from build123d import *

# Parameters (mm, degrees)
F1_R      = 60.325
F2_DEPTH  = 127
F0_R      = 53.975
F3_DEPTH  = 184.912
F5_DEPTH  = 19.05
F6_R      = 1.5875
F7_DEPTH  = 25.4
F8_R      = 1.5875
F9_DEPTH  = 25.4
F10_R     = 1.5875
F11_DEPTH = 36.6522


with BuildPart() as f2:
    # F1 (on Top) → F2 (new body)
    with BuildSketch(Plane.XY):
        Circle(F1_R)
    extrude(amount=F2_DEPTH)

    # F0 (on Top) → F3 (cut)
    with BuildSketch(Plane.XY):
        Circle(F0_R)
    extrude(amount=F3_DEPTH, mode=Mode.SUBTRACT)

    # F4 (on Top) → F5 (join)
    with BuildSketch(Plane.XY):
        with BuildLine():
            ThreePointArc((-56.3123252778, 21.5134135298), (-55.0938321912, 24.4657841564), (-53.7206778829, 27.3494736274))
            Line((-53.7206778829, 27.3494736274), (-67.5786357684, 35.350369343))
            Line((-67.5786357684, 35.350369343), (-70.7536357684, 29.851108029))
            Line((-70.7536357684, 29.851108029), (-56.3123252778, 21.5134135298))
        make_face()
        with BuildLine():
            Line((-64.4036357684, 40.849630657), (-50.5456778829, 32.8487349414))
            ThreePointArc((-50.5456778829, 32.8487349414), (-48.7349066985, 35.4797661912), (-46.7873252778, 38.0111974719))
            Line((-46.7873252778, 38.0111974719), (-61.2286357684, 46.348891971))
            Line((-61.2286357684, 46.348891971), (-64.4036357684, 40.849630657))
        make_face()
        with BuildLine():
            Line((67.5786357684, 35.350369343), (53.7206778829, 27.3494736274))
            ThreePointArc((53.7206778829, 27.3494736274), (55.0938321912, 24.4657841564), (56.3123252778, 21.5134135298))
            Line((56.3123252778, 21.5134135298), (70.7536357684, 29.851108029))
            Line((70.7536357684, 29.851108029), (67.5786357684, 35.350369343))
        make_face()
        with BuildLine():
            ThreePointArc((46.7873252778, 38.0111974719), (48.7349066985, 35.4797661912), (50.5456778829, 32.8487349414))
            Line((50.5456778829, 32.8487349414), (64.4036357684, 40.849630657))
            Line((64.4036357684, 40.849630657), (61.2286357684, 46.348891971))
            Line((61.2286357684, 46.348891971), (46.7873252778, 38.0111974719))
        make_face()
        with BuildLine():
            Line((-3.175, -76.2), (-3.175, -60.1982085688))
            ThreePointArc((-3.175, -60.1982085688), (-6.3589254926, -59.9455503476), (-9.525, -59.5246110016))
            Line((-9.525, -59.5246110016), (-9.525, -76.2))
            Line((-9.525, -76.2), (-3.175, -76.2))
        make_face()
        with BuildLine():
            ThreePointArc((9.525, -59.5246110016), (6.3589254926, -59.9455503476), (3.175, -60.1982085688))
            Line((3.175, -60.1982085688), (3.175, -76.2))
            Line((3.175, -76.2), (9.525, -76.2))
            Line((9.525, -76.2), (9.525, -59.5246110016))
        make_face()
    extrude(amount=F5_DEPTH)

    # F6 (on face) → F7 (cut)
    with BuildSketch(Plane(origin=(4.7625, 8.248891971, 0), x_dir=(-0.8660254038, 0.5, 0), z_dir=(0.5, 0.8660254038, 0))):
        with Locations((69.85, 9.525)):
            Circle(F6_R)
    extrude(amount=-F7_DEPTH, mode=Mode.SUBTRACT)

    # F8 (on face) → F9 (cut)
    with BuildSketch(Plane(origin=(4.7625, -8.248891971, 0), x_dir=(0.8660254038, 0.5, 0), z_dir=(0.5, -0.8660254038, 0))):
        with Locations((69.85, 9.525)):
            Circle(F8_R)
    extrude(amount=-F9_DEPTH, mode=Mode.SUBTRACT)

    # F10 (on face) → F11 (cut)
    with BuildSketch(Plane(origin=(-9.525, 0, 0), x_dir=(0, -1, 0), z_dir=(-1, 0, 0))):
        with Locations((69.85, 9.525)):
            Circle(F10_R)
    extrude(amount=-F11_DEPTH, mode=Mode.SUBTRACT)


solid = f2.part
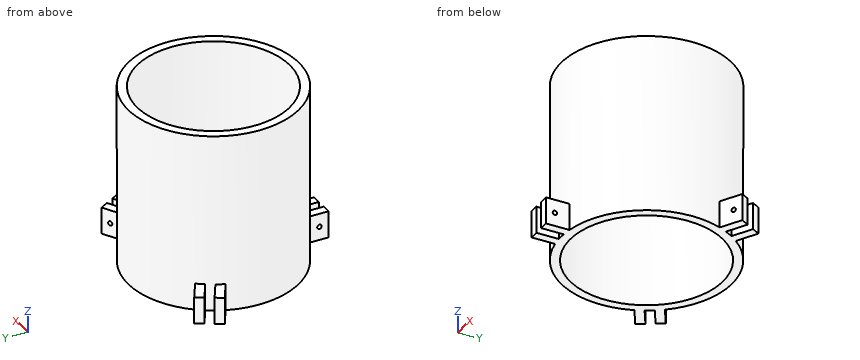
Geometry check sheet. Reference: the model listing, model coordinates, mm. Coordinates: 2 decimals unless noted, no trailing zeros. Order: outer loops, then holes, each group sorted by start corner. A loop starts at its lowest first (then second) coordinate and runs counter-clockwise, first axis right, second up. Notation, with made-up numbers: (10, -33) -> (57, -33) arc R18 cw to (57, -17) -> close; hole circle Ø1 at (-9.75, 57). An arc over 180 degrees is marked (long way). Use a Markdown table: item, result. Add a question column.
1. Cross-section at C-C (z = 88.5). Enter the section's corners in (x, y) (3 decimals), and give its area (3 significant figures).
2. Material ranges on L1, parallel to Y at x = 0, z = 100 (3 decimals); L2, parallel to Z at x = 7.25, y = -69.85; L3, parallel to X at y = -2, z = 97, recorded low to high.
3. Cross-section at A-A (x = 0). Enter the section's corners in (y, z) (3 decimals).
4. Go/stop test with flat-tipped pins: pin 1 Ø8 at (y, z) = (-69, 7.5) entering from -X (3 decimals); pin 2 Ø4 at (y, z) = (-16, 104) entering from +X; pin 3 Ø6.5 at (x, y) = (-57.5, 38.5) entering from +Z. Record where each tip stops, or that it passes through.
Filled sheet:
| question | item | result |
|---|---|---|
| 1 | outline | circle Ø120.65 at (0, 0); hole circle Ø107.95 at (0, 0) |
| 1 | area | 2,280 mm2 |
| 2 | L1 | -60.325 to -53.975, 53.975 to 60.325 |
| 2 | L2 | 0 to 7.94, 11.11 to 19.05 |
| 2 | L3 | -60.29 to -53.94, 53.94 to 60.29 |
| 3 | outline | (-60.325, 0) -> (-53.975, 0) -> (-53.975, 127) -> (-60.325, 127) -> close; (53.975, 0) -> (60.325, 0) -> (60.325, 127) -> (53.975, 127) -> close |
| 4 | pin 1 | x = -9.525 |
| 4 | pin 2 | x = 58.68 |
| 4 | pin 3 | z = 19.05 |
